from build123d import *

# Parameters (mm, degrees)
F1_DEPTH = 100
F2_T     = -1
F5_D     = 20


# Not quite as in the source:
# - the program builds the solid bodies; features that only make, move or delete a surface that nothing else refers to are left out


with BuildPart() as f1:
    # F0 (on Front) → F1 (new body)
    with BuildSketch(Plane.XZ):
        Polygon((0, 200), (0, 0), (400, 0), (1200, 400), (1600, 400), (1600, 600), (1200, 600), (400, 200), align=None)
    extrude(amount=F1_DEPTH)

    # F2
    f2_openings = [f1.faces().sort_by_distance(p)[0] for p in [
        (200, -50, 200),
        (800, -50, 400),
        (1400, -50, 600),
    ]]
    offset(amount=F2_T, openings=f2_openings, kind=Kind.INTERSECTION)

    # F5 (through all)
    with Locations(Plane.XY.offset(401)):
        with Locations((1587, -13), (1587, -87)):
            Hole(F5_D / 2)


solid = f1.part
Check sheet for the modelled part. Datum: model origin and axes. Units: mm. A direction names the side the tool comes from. Give positions to 0.01 mm unless a question says otherwise; leave off trailing zeros. Write each loop counter-clockwise with the first axis right and the second up, starting at its lowest first coordinate (ties: lowest second). Pieces come first, ordered by that corner, then holes. Notation, with made-up numbers: (13, -38) -> (42, -38) arc R18 ccw to (42, -28) -> close; hole circle Ø6 at (23.5, 50). An arc over 180 degrees is marked (long way). One line per item, written item: value. Start each with the question number.
Item 1: Section check C-C on z = 53.5. Record the cut outline in (x, y), then the cut area to 3 significant figures.
Item 2: Section check B-B on x = 1497. Record the cut outline in (y, z).
Item 3: Draft check along Y on faces 4 (the flat face through (796, 0, 324)), 5 (the flat face through (805.6, -0.5, 402.8)), 6 (the flat face through (198, -49, 1)). Enter one of: +Y half, -Y half, draft (parallel to the pull), parting line (faces both ways), or undercut.
Item 4: Section check D-D on z = 442.5. Record the cut outline in (x, y).
Item 5: Section check A-A on y = -47. Record the cut outline in (x, z), then the cut area to 3 significant figures.
Item 6: Tool access check on faces 1 (the flat face through (1397, -49, 400)), 2 (the flat face through (1397, -49, 401)), 3 (the flat face through (794.16, -49.31, 198.2)). Record the directions out of +Z, -Z, +X, -X, +Y, -Y that give a thin tool (end or side, any length) a straight path to the whole face; none if there is none.
Item 7: Gauge pin test, flat ends, axial feed: pin 1 (8 mm diameter, centred on x = 864.5, y = -23, fed in from +Z); pin 2 (10 mm diameter, centred on x = 656, y = -13, fed in from -Z); pin 3 (8 mm diameter, centred on y = -41.5, z = 378.5, fed in from +X). Record the tip position at first contact, or that the pin passes through.
Item 8: Material ranges on probe 1 along Y at (x, z) = (1587, 400.7); probe 2 along Y at (x, z) = (693, 245.5); probe 3 along Z at (x, y) = (206, -27), recorded low to high. Write a range as from..to.
Results list:
1. outline: (0, -100) -> (507, -100) -> (507, 0) -> (0, 0) -> close; hole (1, -99) -> (504.76, -99) -> (504.76, -1) -> (1, -1) -> close
1. area: 1,330 mm²
2. outline: (-100, 400) -> (0, 400) -> (0, 600) -> (-1, 600) -> (-1, 401) -> (-99, 401) -> (-99, 600) -> (-100, 600) -> close
3. face 4: +Y half
3. face 5: draft
3. face 6: undercut
4. outline: (885, -100) -> (1600, -100) -> (1600, 0) -> (885, 0) -> (885, -1) -> (1599, -1) -> (1599, -99) -> (885, -99) -> close
5. outline: (0, 0) -> (400, 0) -> (1200, 400) -> (1600, 400) -> (1600, 600) -> (1599, 600) -> (1599, 401) -> (1199.76, 401) -> (399.76, 1) -> (1, 1) -> (1, 200) -> (0, 200) -> close
5. area: 2,090 mm²
6. face 1: -Z, +X, +Y, -Y
6. face 2: +Z, -X
6. face 3: +Z
7. pin 1: z = 235.37
7. pin 2: z = 125.5
7. pin 3: x = 1165
8. probe 1: -100..-97, -77..-23, -3..0
8. probe 2: -100..-99, -1..0
8. probe 3: 0..1
